Geometry: see drawing. Coordinates: mm, zero at the bounding-box minimum. A direction names the side the tool comes from. Coordinates: 2 decimals unless noted, no trailing zeros. Loops run counter-clockwise (first coordinate to the right, second up) from the corner with the lowest first, then second, coordinate; pieces in that order, holes last. Notation, with made-up numbers: (71, 29) - (80, 29) arc R10 cw to (80, 42) - close; hole circle Ø2 at (-26.75, 17). An arc over 180 degrees is marked (long way). Use one line per item in the form item = value.
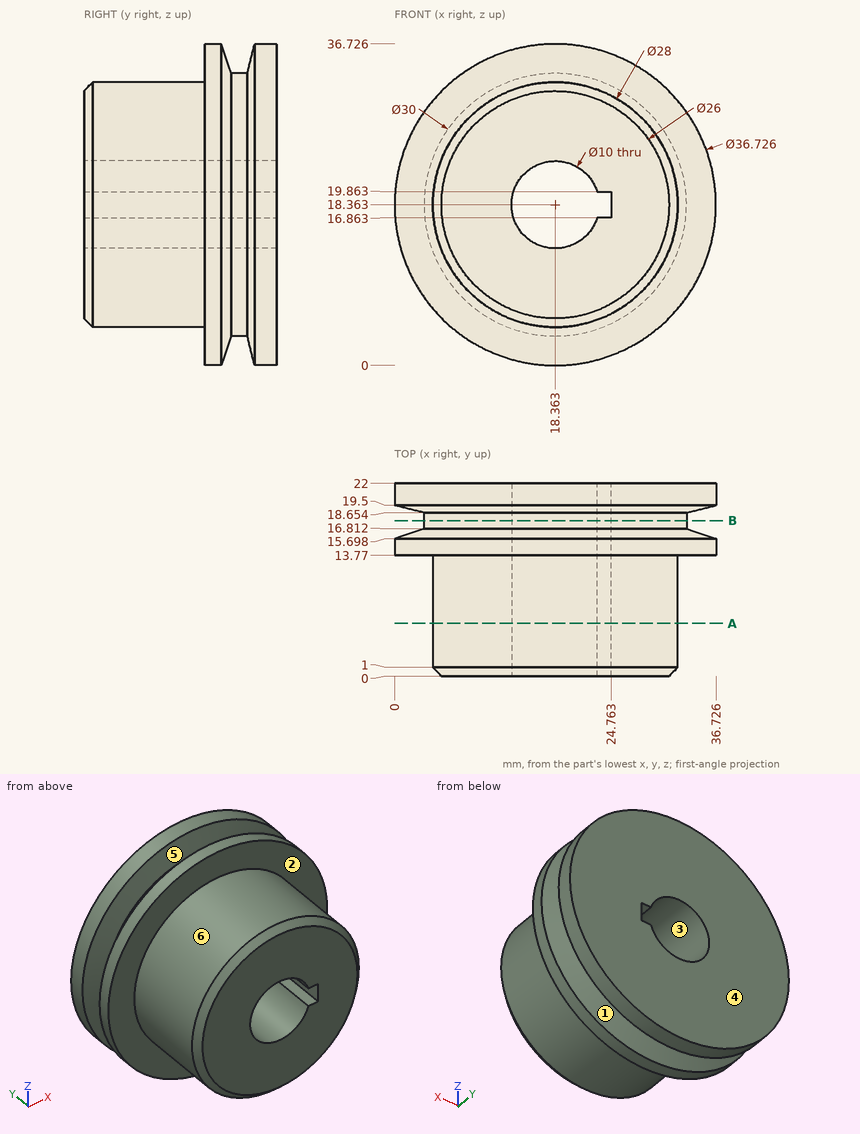
Q1. Cut plane A-A, the plane y = 6. Return loops of the section in (x, z), then the cut area to 3 significant figures.
Check values:
outline = circle Ø28 at (18.36, 18.36); hole (23.13, 16.86) - (24.76, 16.86) - (24.76, 19.86) - (23.13, 19.86) arc R5 ccw (long way) to start
area = 533 mm²
Q2. First-contact query: P1, Ø1, axis at y = 6.5, z = 31.5, coming from the +X side (1 decimal); P2, Ø5, axis at y = 8, z = 31.5, coming from the +X side (1 decimal); P3, Ø3.5, axis at y = 9, z = 18.5, coming from the -X side; P4, Ø10, axis at x = 22, z = 20.5, coming from the -Y side. Flat tips, straight axial feed; report the tip coordinate or a pass-through.
Check values:
P1 = 24.4
P2 = 27.5
P3 = 4.36
P4 = 0
Q3. Ray query, line 1 along Y through (x, z) = (12.5, 35); line 2 along Z through (x, y) = (16, 21) (1 decimal); line 3 along Y through (x, z) = (2, 24.5). Return the intervals inside material, ascending. Write a range as [from, to].
Check values:
line_1 = [13.77, 15.94], [19.32, 22]
line_2 = [0.2, 14], [22.8, 36.6]
line_3 = [13.77, 15.99], [19.28, 22]
Q4. Cut plane B-B, the plane y = 17.75. Return loops of the section in (x, z).
Check values:
outline = circle Ø30 at (18.36, 18.36); hole (23.13, 16.86) - (24.76, 16.86) - (24.76, 19.86) - (23.13, 19.86) arc R5 ccw (long way) to start
Q5. Pull-direction query (X, two-part tool) for the marked faces 1, 2 and 3; classes: pulls with the +X half, pulls with the -X half, needs draft (parallel to the pull), parting line crosses it, or undercut.
Check values:
face_1 = parting line crosses it
face_2 = needs draft
face_3 = undercut
Q6. Set-up query: the marked faces 4, 5 and 6. Return all of +Z, -Z, +X, -X, +Y, -Y with unobstructed straight access to the full face (end or side cutting, diameter ignored); none if empty.
Check values:
face_4 = +Z, -Z, +X, -X, +Y
face_5 = none
face_6 = -Y
